The drawing under review shows one solid part. Ordinate dimensions are in mm from its lowest x, y, z. Coordinates: 2 decimals unless noted, no trailing zeros. Loops run counter-clockwise (first coordinate to the right, second up) from the corner with the lowest first, then second, coordinate; pieces in that order, holes last. Notation, with made-up numbers: M 84,65.25 L 127,65.25 A9 ccw 127,71.25 Z; hole C -33.5,6 d1. An arc over 180 degrees is marked long. Answer as a JSON object with one key per item and string values. Group by question number.
1. Consider section B-B (z = 17.5). State the section outline as (x, y) points, then the cut area to 3 significant figures.
2. Draft analysis for pull direction X (two halves, no side actions). For the marked faces 1, 2 and 3, state which applies: +X half, -X half, draft (parallel to the pull), parting line (faces both ways), or undercut.
3. Consider section C-C (x = 106.68). State the section outline as (y, z) points (1 decimal).
4. Consider section A-A (y = 28). Count the separate pieces of the cut face and the enclosed holes in it, then the cut area to 3 significant figures.
5. To check wall thickness, follow probe 1 along X at (y, z) = (28, 16.75) (1 decimal); probe 2 along Z at (x, y) = (144.78, 31); probe 3 along X at (y, z) = (29, 16.25) (1 decimal). State the ranges of each line that lie inside material, in increasing order.
6. Insertion check: pin 1 (12 mm diameter, centred on y = 36.5, z = 3, fed in from -X); pin 2 (7.5 mm diameter, centred on x = 75, z = 13.5, fed in from -Y); pin 3 (1 mm diameter, centred on x = 108, y = 15, fed in from -Z). Each pin has a flat end and moves straight along its axis. Give the tip position at first contact, or say it passes through.
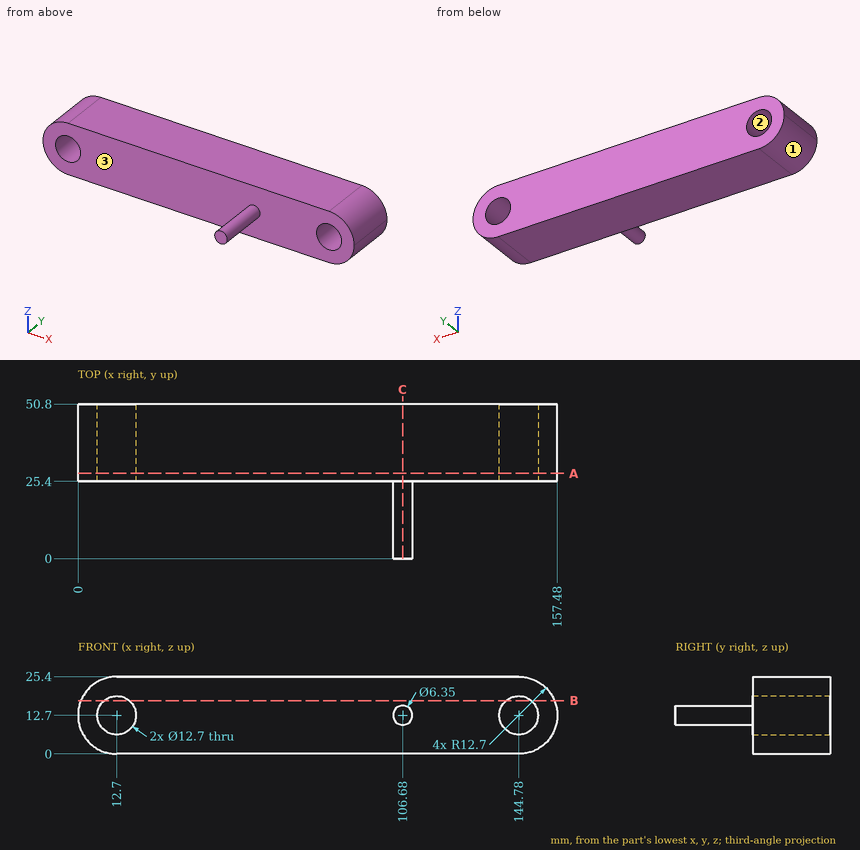
Findings below:
{
 "1": {"outline": "M 0.94,25.4 L 8.54,25.4 L 8.54,50.8 L 0.94,50.8 Z; M 16.86,25.4 L 140.62,25.4 L 140.62,50.8 L 16.86,50.8 Z; M 148.94,25.4 L 156.54,25.4 L 156.54,50.8 L 148.94,50.8 Z", "area": "3,530 mm^2"},
 "2": {"face 1": "-X half", "face 2": "undercut", "face 3": "draft"},
 "3": {"outline": "M 0,9.5 L 25.4,9.5 L 25.4,0 L 50.8,0 L 50.8,25.4 L 25.4,25.4 L 25.4,15.9 L 0,15.9 Z"},
 "4": {"separate pieces": "1", "enclosed holes": "2", "area": "3,610 mm^2"},
 "5": {"probe 1": "x = 0.7 to 7.8, 17.6 to 139.9, 149.7 to 156.8", "probe 2": "z = 0 to 6.35, 19.05 to 25.4", "probe 3": "x = 0.5 to 7.4, 18 to 139.5, 150 to 157"},
 "6": {"pin 1": "stops at x = 0.55", "pin 2": "stops at y = 25.4", "pin 3": "stops at z = 9.63"}
}
